Autodesk Fusion 360 part; units mm, degrees
sketch "Szkic1" plane through (0, 0, 0) normal (0, 0, 1) x (1, 0, 0)
  line L0 (0, 0) -> (100, 0)
  line L1 (100, 0) -> (100, 100)
  line L2 (100, 100) -> (0, 100)
  line L3 (0, 100) -> (0, 0)
  dimension "d1" = 100
  dimension "d2" = 100
extrude "Wyciągnięcie proste1" add sketch "Szkic1" along normal blind 3
sketch "Szkic2" plane through (0, 0, 3) normal (0, 0, 1) x (-1, 0, 0)
  line L0 (0, -100) -> (0, 0)
  line L1 (0, 0) -> (-100, 0)
  line L2 (-100, 0) -> (-100, -100)
  line L3 (-100, -100) -> (0, -100)
  line L4 (-10, -10) -> (-90, -10)
  line L5 (-90, -10) -> (-90, -90)
  line L6 (-90, -90) -> (-10, -90)
  line L7 (-10, -90) -> (-10, -10)
extrude "Wyciągnięcie proste2" cut sketch "Szkic2" against normal blind 3 contours L4 L5 L6 L7
sketch "Szkic3" plane through (0, 0, 3) normal (0, 0, 1) x (-1, 0, 0)
  line L0 (-90, -10) -> (-10, -10)
  line L1 (-10, -10) -> (-10, -90)
  line L2 (-10, -90) -> (-90, -90)
  line L3 (-90, -90) -> (-90, -10)
  line L4 (0, -100) -> (0, 0)
  line L5 (0, 0) -> (-100, 0)
  line L6 (-100, 0) -> (-100, -100)
  line L7 (-100, -100) -> (0, -100)
  line L8 (0, 0) -> (-100, 0)
  line L9 (-100, 0) -> (-100, -3)
  line L10 (-100, -3) -> (0, -3)
  line L11 (0, -3) -> (0, 0)
  line L12 (-100, -3) -> (-96.5907, -3)
  line L13 (-96.5907, -3) -> (-96.5907, -100)
  line L14 (-96.5907, -100) -> (-100, -100)
  line L15 (-100, -100) -> (-100, -3)
  line L16 (-96.5907, -100) -> (0, -100)
  line L17 (0, -100) -> (0, -97)
  line L18 (0, -97) -> (-96.5907, -97)
  line L19 (-96.5907, -97) -> (-96.5907, -100)
extrude "Wyciągnięcie proste3" add sketch "Szkic3" along normal blind 20 contours L4 L7 L13 L16 L17 L18 L19 | L6 L7 L10 L12 L13 L14 L15 L19 | L4 L5 L6 L8 L9 L10 L11 L12
sketch "Szkic4" plane through (0, 0, 3) normal (0, 0, 1) x (-1, 0, 0)
  line L0 (0, -3) -> (-96.5907, -3)
  line L1 (-96.5907, -3) -> (-96.5907, -97)
  line L2 (-96.5907, -97) -> (0, -97)
  line L3 (0, -97) -> (0, -3)
  line L4 (-90, -10) -> (-10, -10)
  line L5 (-10, -10) -> (-10, -90)
  line L6 (-10, -90) -> (-90, -90)
  line L7 (-90, -90) -> (-90, -10)
  line L8 (0, -97) -> (0, -89)
  line L9 (0, -89) -> (2, -89)
  line L10 (2, -89) -> (2, -91)
  line L11 (2, -91) -> (6, -91)
  line L12 (0, -89) -> (0, -83)
  line L13 (2, -83) -> (2, -81)
  line L14 (2, -81) -> (6, -81)
  line L15 (6, -81) -> (6, -91)
  line L16 (2, -83) -> (0, -83)
  line L17 (0, -83) -> (0, -89.2495)
extrude "Wyciągnięcie proste4" add sketch "Szkic4" against normal blind 3 contours L3 L9 L10 L11 L12 L13 L14 L15 L16 L17
sketch "Szkic5" plane through (0, 0, 23) normal (0, 0, 1) x (-1, 0, 0)
  line L0 (-100, -100) -> (0, -100)
  line L1 (0, -100) -> (0, -97)
  line L2 (0, -97) -> (-96.5907, -97)
  line L3 (-96.5907, -97) -> (-96.5907, -3)
  line L4 (-96.5907, -3) -> (0, -3)
  line L5 (0, -3) -> (0, 0)
  line L6 (0, 0) -> (-100, 0)
  line L7 (-100, 0) -> (-100, -100)
  line L8 (-45, -100) -> (-55, -100)
  line L9 (-55, -100) -> (-55, -110)
  line L10 (-55, -110) -> (-45, -110)
  line L11 (-45, -110) -> (-45, -100)
  line L12 (-100, -55) -> (-110, -55)
  line L13 (-110, -55) -> (-110, -45)
  line L14 (-110, -45) -> (-100, -45)
  line L15 (-100, -45) -> (-100, -55)
  line L16 (-45, 0) -> (-55, 0)
  line L17 (-55, 0) -> (-55, 10)
  line L18 (-55, 10) -> (-45, 10)
  line L19 (-45, 10) -> (-45, 0)
extrude "Wyciągnięcie proste5" add sketch "Szkic5" against normal blind 2 contours L0 L8 L9 L10 L11 | L7 L12 L13 L14 L15 | L6 L16 L17 L18 L19
sketch "Szkic6" plane through (45, 0, 0) normal (-1, 0, 0) x (0, -1, 0)
  line L0 (10, 23) -> (0, 23)
  line L1 (0, 23) -> (0, 21)
  line L2 (0, 21) -> (10, 21)
  line L3 (10, 21) -> (10, 23)
  line L4 (0, 21) -> (0, 18)
  line L5 (0, 18) -> (10, 21)
  line L6 (0, 21) -> (10, 21)
extrude "Wyciągnięcie proste6" add sketch "Szkic6" against normal blind 10 contours L2 L4 L5 L6
sketch "Szkic7" plane through (0, 45, 0) normal (0, -1, 0) x (1, 0, 0)
  line L0 (110, 23) -> (100, 23)
  line L1 (100, 23) -> (100, 21)
  line L2 (100, 21) -> (110, 21)
  line L3 (110, 21) -> (110, 23)
  line L4 (100, 21) -> (100, 18)
  line L5 (100, 18) -> (110, 21)
  line L6 (100, 21) -> (110, 21)
extrude "Wyciągnięcie proste7" add sketch "Szkic7" against normal blind 10 contours L2 L4 L5 L6
sketch "Szkic8" plane through (55, 0, 0) normal (1, 0, 0) x (0, 1, 0)
  line L0 (110, 23) -> (100, 23)
  line L1 (100, 23) -> (100, 21)
  line L2 (100, 21) -> (110, 21)
  line L3 (110, 21) -> (110, 23)
  line L4 (100, 21) -> (100, 18)
  line L5 (100, 18) -> (110, 21)
  line L6 (100, 21) -> (110, 21)
extrude "Wyciągnięcie proste8" add sketch "Szkic8" against normal blind 10 contours L2 L4 L5 L6
sketch "Szkic9" plane through (0, 0, 23) normal (0, 0, 1) x (-1, 0, 0)
  line L0 (-100, -100) -> (-55, -100)
  line L1 (-55, -100) -> (-55, -110)
  line L2 (-55, -110) -> (-45, -110)
  line L3 (-45, -110) -> (-45, -100)
  line L4 (-45, -100) -> (0, -100)
  line L5 (0, -100) -> (0, -97)
  line L6 (0, -97) -> (-96.5907, -97)
  line L7 (-96.5907, -97) -> (-96.5907, -3)
  line L8 (-96.5907, -3) -> (0, -3)
  line L9 (0, -3) -> (0, 0)
  line L10 (0, 0) -> (-45, 0)
  line L11 (-45, 0) -> (-45, 10)
  line L12 (-45, 10) -> (-55, 10)
  line L13 (-55, 10) -> (-55, 0)
  line L14 (-55, 0) -> (-100, 0)
  line L15 (-100, 0) -> (-100, -45)
  line L16 (-100, -45) -> (-110, -45)
  line L17 (-110, -45) -> (-110, -55)
  line L18 (-110, -55) -> (-100, -55)
  line L19 (-100, -55) -> (-100, -100)
  circle A0 centre (-50, 5) radius 2.5
  circle A1 centre (-105, -50) radius 2.5
  circle A2 centre (-50, -105) radius 2.5
  dimension "d19" = 5
  dimension "d20" = 5
  dimension "d21" = 5
extrude "Wyciągnięcie proste9" cut sketch "Szkic9" against normal blind 2 contours A0 | A1 | A2
Geometry check sheet. Reference: the model listing, model coordinates, mm. A direction names the side the tool comes from. Give positions to 0.01 mm unless a question says otherwise; leave off trailing zeros. Loops run counter-clockwise (first coordinate to the right, second up) from the corner with the lowest first, then second, coordinate; pieces in that order, holes last. Notation, with made-up numbers: M 43.25,68.25 L 55.25,68.25 A12 cw 55.25,79.25 Z; hole C -12.5,20 d2. An arc over 180 degrees is marked long. Answer as a JSON object with one key per item and string values. Group by question number.
Item 1: Mould release check, pull along Y, two halves, no side actions. Record for faces 1 (the flat face through (50.07, 104.93, 19.48)), 2 (the flat face through (96.591, 49, 13)), 3 (the flat face through (100, 49, 11)): pulls with the +Y half, pulls with the -Y half, needs draft (parallel to the pull), parting line crosses it, or undercut.
Item 2: Material ranges on L1, parallel to Y at x = 50, z = 22.3; L2, parallel to Y at x = 16.5, z = 2; L3, parallel to Y at x = 76.5, z = 10.75, recorded low to high.
Item 3: Gauge pin test, flat ends, axial feed: pin 1 (12 mm diameter, centred on x = 72.5, y = 18, fed in from -Z); pin 2 (0.9 mm diameter, centred on x = 34.5, z = 2, fed in from -Y); pin 3 (10 mm diameter, centred on y = 53, z = 17, fed in from -X); pin 4 (1.5 mm diameter, centred on x = 103.5, z = 21, fed in from -Y). Record the tip position at first contact, or that the pin passes through.
Item 4: Sectioned sample at B-B on x = 50. Record the boundary of the cut face in (y, z), plus the area to 3 significant figures.
Item 5: Sectioned sample at A-A on y = 50. Record the boundary of the cut face in (x, z).
Item 6: Access from +Z, -Z, +X, -X, +Y, -Y to the whole of each face (thin tool, end or side, straight path). Record for faces 4 (the flat face through (-4, 81, 2)), 5 (the flat face through (55, -4, 21)), 6 (the flat face through (90, 49, 2)), 7 (the flat face through (48, 97, 13)), 8 (the flat face through (50, 105, 21)).
Item 7: Sectioned sample at D-D on z = 5.25. Record the boundary of the cut face in (x, y).
Item 8: Sectioned sample at C-C on y = 105. Record the boundary of the cut face in (x, z), plus the area to 3 significant figures.
Findings below:
{
 "1": {"face 1": "pulls with the +Y half", "face 2": "undercut", "face 3": "needs draft"},
 "2": {"L1": "-10 to -7.5, -2.5 to 3, 97 to 102.5, 107.5 to 110", "L2": "0 to 10, 90 to 100", "L3": "0 to 3, 97 to 100"},
 "3": {"pin 1": "through", "pin 2": "y = 0", "pin 3": "x = 96.59", "pin 4": "y = 45"},
 "4": {"outline": "M -10,21 L 0,18 L 0,0 L 10,0 L 10,3 L 3,3 L 3,23 L -2.5,23 L -2.5,21 L -7.5,21 L -7.5,23 L -10,23 Z; M 90,0 L 100,0 L 100,18 L 110,21 L 110,23 L 107.5,23 L 107.5,21 L 102.5,21 L 102.5,23 L 97,23 L 97,3 L 90,3 Z", "area": "230 mm2"},
 "5": {"outline": "M 0,0 L 10,0 L 10,3 L 0,3 Z; M 90,0 L 100,0 L 100,18 L 110,21 L 110,23 L 107.5,23 L 107.5,21 L 102.5,21 L 102.5,23 L 96.59,23 L 96.59,3 L 90,3 Z"},
 "6": {"face 4": "+Z, -Z, -X, -Y", "face 5": "+Z, -Z, +X, -Y", "face 6": "+Z, -Z", "face 7": "+Z, -X", "face 8": "+Z"},
 "7": {"outline": "M 0,0 L 100,0 L 100,100 L 0,100 L 0,97 L 96.59,97 L 96.59,3 L 0,3 Z"},
 "8": {"outline": "M 45,19.5 L 55,19.5 L 55,23 L 52.5,23 L 52.5,21 L 47.5,21 L 47.5,23 L 45,23 Z", "area": "25.0 mm2"}
}
